Design review of the part shown in the three views and the two pictorial views. Dimensions are in mm from the part's minimum x, y and z. Coordinates: 2 decimals unless noted, no trailing zeros. Loops run counter-clockwise (first coordinate to the right, second up) from the corner with the lowest first, then second, coordinate; pieces in that order, holes last. Notation, with made-up numbers: (6.5, -2) -> (40.5, -2) arc R26 ccw to (40.5, 30) -> close; hole circle Ø9 at (-37, -39.75). An arc over 180 degrees is marked (long way). One line per item, written item: value. Start each with the question number.
1. Insertion check: pin 1 (5.5 mm diameter, centred on x = 29.925, z = 4.2, fed in from -Y); pin 2 (0.7 mm diameter, centred on y = 1, z = 64.5, fed in from +X) (3 decimals); pin 3 (3 mm diameter, centred on x = 22.075, z = 4.2, fed in from -Y). Each pin has a flat end and moves straight along its axis. Give the tip position at first contact, or say it passes through.
2. For probe 1 along X at (y, z) = (0.5, 4.2) (3 decimals); probe 2 along X at (y, z) = (0.85, 3); probe 3 along Z at (x, y) = (36, 0.8), list the stretches that pass through material, from the lowest coordinate up.
3. Add section B-B on y = 1.1. Write out the cut boundary in (x, z) (3 decimals), plus the area to 3 significant figures.
4. Add section C-C on x = 49. Write out the cut boundary in (y, z) (3 decimals).
5. Add section D-D on x = 15.5. Write out the cut boundary in (y, z), plus the area to 3 significant figures.
6. Add section A-A on z = 4.2. Write out the cut boundary in (x, y) (3 decimals), plus the area to 3 significant figures.
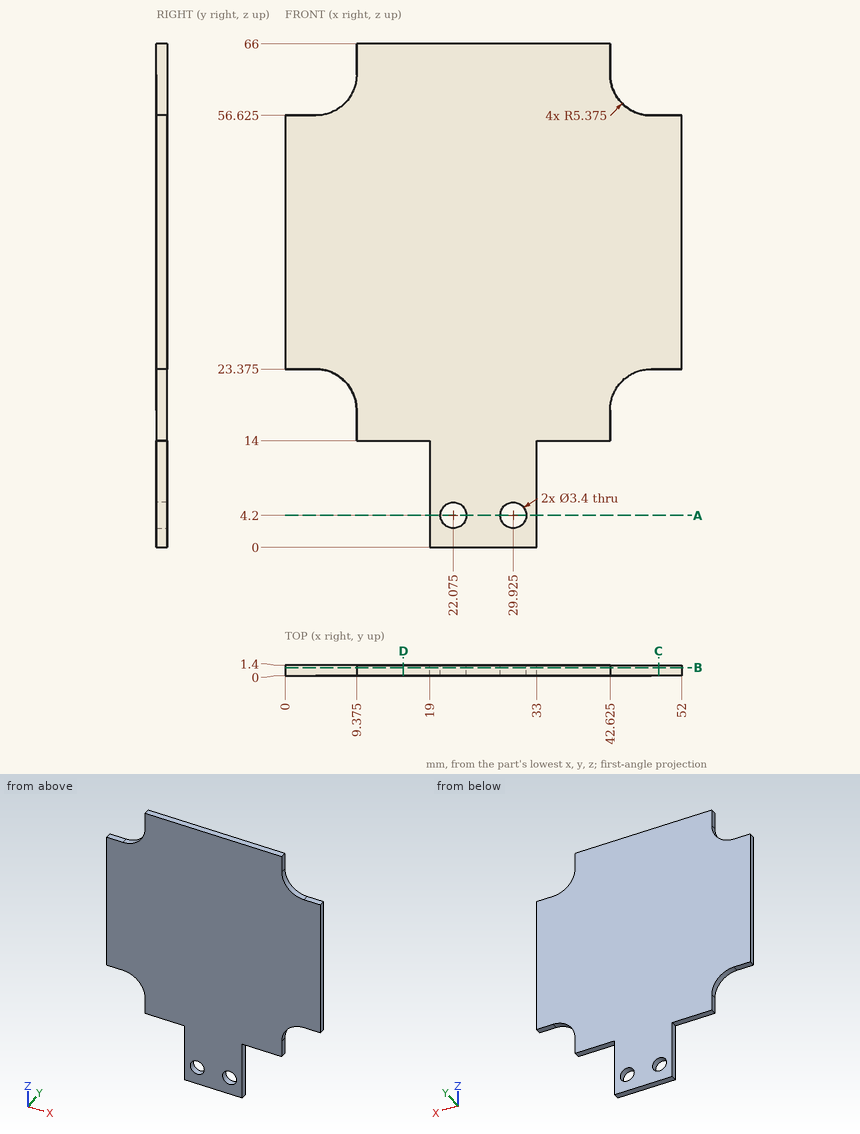
Worked answers:
1. pin 1: stops at y = 0
1. pin 2: stops at x = 42.625
1. pin 3: passes through
2. probe 1: x = 19 to 20.375, 23.775 to 28.225, 31.625 to 33
2. probe 2: x = 19 to 20.87, 23.28 to 28.72, 31.13 to 33
2. probe 3: z = 14 to 66
3. outline: (0, 23.375) -> (4, 23.375) arc R5.375 cw to (9.375, 18) -> (9.375, 14) -> (19, 14) -> (19, 0) -> (33, 0) -> (33, 14) -> (42.625, 14) -> (42.625, 18) arc R5.375 cw to (48, 23.375) -> (52, 23.375) -> (52, 56.625) -> (48, 56.625) arc R5.375 cw to (42.625, 62) -> (42.625, 66) -> (9.375, 66) -> (9.375, 62) arc R5.375 cw to (4, 56.625) -> (0, 56.625) -> close; hole circle Ø3.4 at (22.075, 4.2); hole circle Ø3.4 at (29.925, 4.2)
3. area: 2,560 mm²
4. outline: (0, 23.375) -> (1.4, 23.375) -> (1.4, 56.625) -> (0, 56.625) -> close
5. outline: (0, 14) -> (1.4, 14) -> (1.4, 66) -> (0, 66) -> close
5. area: 72.8 mm²
6. outline: (19, 0) -> (20.375, 0) -> (20.375, 1.4) -> (19, 1.4) -> close; (23.775, 0) -> (28.225, 0) -> (28.225, 1.4) -> (23.775, 1.4) -> close; (31.625, 0) -> (33, 0) -> (33, 1.4) -> (31.625, 1.4) -> close
6. area: 10.1 mm²
